Autodesk Inventor part; units mm, degrees
ref_plane "YZ Plane" through (0, 0, 0) normal (1, 0, 0) x (0, 1, 0)
ref_plane "XZ Plane" through (0, 0, 0) normal (0, 1, 0) x (-1, 0, 0)
ref_plane "XY Plane" through (0, 0, 0) normal (0, 0, 1) x (1, 0, 0)
sketch "Sketch1" plane through (0, 0, 0) normal (0, 0, 1) x (1, 0, 0)
  circle A0 centre (0, 0) radius 17.5
  line L0 (14.8492, -14.8492) -> (-14.8492, -14.8492) construction
  line L1 (-14.8492, -14.8492) -> (-14.8492, 14.8492) construction
  line L2 (-14.8492, 14.8492) -> (14.8492, 14.8492) construction
  line L3 (14.8492, 14.8492) -> (14.8492, -14.8492) construction
  line L4 (14.8492, -14.8492) -> (-14.8492, 14.8492) construction
  line L5 (-14.8492, -14.8492) -> (14.8492, 14.8492) construction
  circle A1 centre (0, 0) radius 21 construction
  line L6 (21, -21) -> (-21, -21) construction
  line L7 (-21, -21) -> (-21, 21) construction
  line L8 (-21, 21) -> (21, 21) construction
  line L9 (21, 21) -> (21, -21) construction
  line L10 (21, -21) -> (-21, 21) construction
  line L11 (-21, -21) -> (21, 21) construction
  line L12 (-31.85, -21.15) -> (-74.15, -21.15) construction
  line L13 (-74.15, -21.15) -> (-74.15, 21.15) construction
  line L14 (-74.15, 21.15) -> (-31.85, 21.15) construction
  line L15 (-31.85, 21.15) -> (-31.85, -21.15) construction
  line L16 (-31.85, -21.15) -> (-74.15, 21.15) construction
  line L17 (-74.15, -21.15) -> (-31.85, 21.15) construction
  line L18 (-37.5, -15.5) -> (-68.5, -15.5) construction
  line L19 (-68.5, -15.5) -> (-68.5, 15.5) construction
  line L20 (-68.5, 15.5) -> (-37.5, 15.5) construction
  line L21 (-37.5, 15.5) -> (-37.5, -15.5) construction
  line L22 (-37.5, -15.5) -> (-68.5, 15.5) construction
  line L23 (-68.5, -15.5) -> (-37.5, 15.5) construction
  line L24 (-70.5, 15.5) -> (-66.5, 15.5) construction
  line L25 (-70.5, 13.85) -> (-66.5, 13.85)
  line L26 (-66.5, 17.15) -> (-70.5, 17.15)
  arc A2 (-70.5, 17.15) -> (-70.5, 13.85) centre (-70.5, 15.5) ccw
  arc A3 (-66.5, 13.85) -> (-66.5, 17.15) centre (-66.5, 15.5) ccw
  line L27 (-35.5, 15.5) -> (-39.5, 15.5) construction
  line L28 (-35.5, 17.15) -> (-39.5, 17.15)
  line L29 (-39.5, 13.85) -> (-35.5, 13.85)
  arc A4 (-35.5, 13.85) -> (-35.5, 17.15) centre (-35.5, 15.5) ccw
  arc A5 (-39.5, 17.15) -> (-39.5, 13.85) centre (-39.5, 15.5) ccw
  line L30 (-35.5, -15.5) -> (-39.5, -15.5) construction
  line L31 (-35.5, -13.85) -> (-39.5, -13.85)
  line L32 (-39.5, -17.15) -> (-35.5, -17.15)
  arc A6 (-35.5, -17.15) -> (-35.5, -13.85) centre (-35.5, -15.5) ccw
  arc A7 (-39.5, -13.85) -> (-39.5, -17.15) centre (-39.5, -15.5) ccw
  line L33 (-70.5, -15.5) -> (-66.5, -15.5) construction
  line L34 (-70.5, -17.15) -> (-66.5, -17.15)
  line L35 (-66.5, -13.85) -> (-70.5, -13.85)
  arc A8 (-70.5, -13.85) -> (-70.5, -17.15) centre (-70.5, -15.5) ccw
  arc A9 (-66.5, -17.15) -> (-66.5, -13.85) centre (-66.5, -15.5) ccw
  line L36 (-55, 0) -> (-51, 0) construction
  line L37 (-55, -11.25) -> (-51, -11.25)
  line L38 (-51, 11.25) -> (-55, 11.25)
  arc A10 (-55, 11.25) -> (-55, -11.25) centre (-55, 0) ccw
  arc A11 (-51, -11.25) -> (-51, 11.25) centre (-51, 0) ccw
  line L39 (40, 54.25) -> (-40, 54.25) construction
  line L40 (-40, 54.25) -> (-40, 94.25) construction
  line L41 (-40, 94.25) -> (40, 94.25) construction
  line L42 (40, 94.25) -> (40, 54.25) construction
  line L43 (40, 54.25) -> (-40, 94.25) construction
  line L44 (-40, 54.25) -> (40, 94.25) construction
  line L45 (98.5, -30) -> (-98.5, -30)
  line L46 (-98.5, -30) -> (-98.5, 30)
  line L47 (-98.5, 30) -> (98.5, 30)
  line L48 (98.5, 30) -> (98.5, -30)
  line L49 (98.5, -30) -> (-98.5, 30) construction
  line L50 (-98.5, -30) -> (98.5, 30) construction
  line L51 (-77, 22) -> (-29, 22)
  line L52 (-29, 22) -> (-29, -22)
  line L53 (-29, -22) -> (-77, -22)
  line L54 (-77, -22) -> (-77, 22)
  line L55 (-77, 22) -> (-29, -22) construction
  line L56 (-29, 22) -> (-77, -22) construction
  line L57 (80, 30) -> (100, 30) construction
  line L58 (100, 30) -> (100, -30) construction
  line L59 (100, -30) -> (80, -30) construction
  line L60 (80, -30) -> (80, 30) construction
  line L61 (80, 30) -> (100, -30) construction
  line L62 (100, 30) -> (80, -30) construction
  line L63 (-80, 30) -> (-100, 30) construction
  line L64 (-100, 30) -> (-100, -30) construction
  line L65 (-100, -30) -> (-80, -30) construction
  line L66 (-80, -30) -> (-80, 30) construction
  line L67 (-80, 30) -> (-100, -30) construction
  line L68 (-100, 30) -> (-80, -30) construction
  line L69 (-83, -28) -> (-23, -28) construction
  line L70 (-23, -28) -> (-23, 28) construction
  line L71 (-23, 28) -> (-83, 28) construction
  line L72 (-83, 28) -> (-83, -28) construction
  circle A12 centre (0, 0) radius 34 construction
  line L73 (-28, -28) -> (28, -28) construction
  line L74 (28, -28) -> (28, 28) construction
  line L75 (28, 28) -> (-28, 28) construction
  line L76 (-28, 28) -> (-28, -28) construction
  line L77 (-28, -28) -> (28, 28) construction
  line L78 (28, -28) -> (-28, 28) construction
  circle A13 centre (0, 0) radius 25 construction
  line L79 (0, 0) -> (9.5671, 23.097) construction
  point P0 (-53, 0)
  point P1 (0, 74.25)
  point P2 (90, 0)
  point P3 (-90, 0)
  dimension "d1" = 42
  dimension "d44" = 50
  dimension "d0" = 35
  dimension "d2" = 42
  dimension "d3" = 42
  dimension "d4" = 42.3
  dimension "d5" = 42.3
  dimension "d6" = 53
  dimension "d7" = 31
  dimension "d8" = 31
  dimension "d9" = 1.65
  dimension "d10" = 4
  dimension "d11" = 11.25
  dimension "d12" = 80
  dimension "d13" = 40
  dimension "d14" = 54.25
  dimension "d15" = 197
  dimension "d16" = 60
  dimension "d35" = 48
  dimension "d36" = 44
  dimension "d37" = 20
  dimension "d38" = 90
  dimension "d39" = 90
  dimension "d40" = 6
  dimension "d41" = 68
  dimension "d42" = 56
  dimension "d43" = 56
  dimension "d45" = 22.5
extrude "Extrusion1" add sketch "Sketch1" along normal blind 6.35 contours L45 L46 L47 L48 | L51 L52 L53 L54
hole "Hole3" at (14.8492, 14.8492, 0) at (-14.8492, 14.8492, 0) at (14.8492, -14.8492, 0) at (-14.8492, -14.8492, 0) direction (0, 0, 1) diameter 3.242 end through all
sketch "Sketch2" plane through (0, 0, 6.35) normal (0, 0, 1) x (1, 0, 0)
  line L0 (90, -21.5) -> (-90, -21.5) construction
  line L1 (-90, -21.5) -> (-90, 21.5) construction
  line L2 (-90, 21.5) -> (90, 21.5) construction
  line L3 (90, 21.5) -> (90, -21.5) construction
  line L4 (90, -21.5) -> (-90, 21.5) construction
  line L5 (-90, -21.5) -> (90, 21.5) construction
  line L6 (98.5, 30) -> (-98.5, 30) construction
  line L7 (-98.5, 30) -> (-90, 30) construction
  line L8 (-90, 30) -> (-90, 21.5) construction
  line L9 (-90, 21.5) -> (-98.5, 21.5) construction
  line L10 (-98.5, 21.5) -> (-98.5, 30) construction
  point P0 (0, 0)
  point P1 (-90, 0)
  point P2 (90, 0)
  dimension "d26" = 180
hole "Hole2" at (-90, 0, 6.35) at (-90, 21.5, 6.35) at (-90, -21.5, 6.35) at (90, 21.5, 6.35) at (90, 0, 6.35) at (90, -21.5, 6.35) direction (0, 0, -1) diameter 5.3 end through all
fillet "Fillet1" radius 2 4 edges at (-98.5, -30, 3.175) (-98.5, 30, 3.175) (98.5, 30, 3.175) (98.5, -30, 3.175)
sketch "Sketch3" plane through (0, 0, 0) normal (0, 0, -1) x (-1, 0, 0)
  line L0 (53, 0) -> (-53, 0) construction
  line L1 (-43, -10) -> (-63, -10) construction
  line L2 (-63, -10) -> (-63, 10) construction
  line L3 (-63, 10) -> (-43, 10) construction
  line L4 (-43, 10) -> (-43, -10) construction
  line L5 (-43, -10) -> (-63, 10) construction
  line L6 (-63, -10) -> (-43, 10) construction
  circle A0 centre (-53, 0) radius 7.5
  point P0 (0, 0)
  point P1 (0, 0)
  dimension "d56" = 20
  dimension "d57" = 20
  dimension "d58" = 15
extrude "Extrusion2" cut sketch "Sketch3" against normal through all
hole "Hole4" at (-53, 0, 0) at (63, 10, 0) at (43, 10, 0) at (43, -10, 0) at (63, -10, 0) direction (0, 0, 1) diameter 3.3 end through all
equation "\"d35\" = d36 + d10"
properties part number "Z-Axis Drive Mount RevII" material "Aluminum 6061"
Work out the finished part from the listing and answer in its coordinate system (mm). A direction names the side the tool comes from. Round coordinates to 2 decimals unless told otherwise and drop trailing zeros. Order: outer loops, then holes, each group sorted by start corner. A loop starts at its lowest first (then second) coordinate and runs counter-clockwise, first axis right, second up. Notation, with made-up numbers: M 28.5,5 L 70.5,5 A6 cw 70.5,13 Z; hole C 19,8 d2. An arc over 180 degrees is marked long. Put each result on its own line as item: value. Start each with the question number.
Q1. Section A-A, the plane y = 0 is taken. Write down the section's boundary in (x, z), and give its area (3 significant figures).
Q2. A tool of negligible diameter and unlimited length cuts with its end or side. For faces 1 (the cylindrical face through (-64.85, 15.54, 3.13)), 2 (the flat face through (98.5, 0, 3)), from which of +Z, -Z, +X, -X, +Y, -Y can it reach the whole face along a straight path? Write none if from no direction.
Q3. Section D-D, the plane y = 21.5 is taken. Write down the section's boundary in (x, z).
Q4. Section B-B, the plane x = 90 is taken. Write down the section's boundary in (y, z).
Q5. For a pull along Y with two mould halves and no side action, classify faces 3 (the flat face through (-1, 30, 3)), 4 (the flat face through (1, -30, 3)), 5 (the cylindrical face through (-13.41, -14.1, 3.22)) as pulls with the +Y half, pulls with the -Y half, needs draft (parallel to the pull), parting line crosses it, or undercut.
Q6. Straight lines are drawn through the part: L1, parallel to Y at x = 63, z = 4.75; L2, parallel to X at y = 21.5, z = 3.5; L3, parallel to X at y = 5, z = 0.75. For each, find the intervals that lie inside material, in ascending order. Write a range as [from, to].
Q7. Section C-C, the plane x = 43 is taken. Write down the section's boundary in (y, z).
Findings below:
1. outline: M -98.5,0 L -92.65,0 L -92.65,6.35 L -98.5,6.35 Z; M -87.35,0 L -66.25,0 L -66.25,6.35 L -87.35,6.35 Z; M -39.75,0 L -17.5,0 L -17.5,6.35 L -39.75,6.35 Z; M 17.5,0 L 45.5,0 L 45.5,6.35 L 17.5,6.35 Z; M 60.5,0 L 87.35,0 L 87.35,6.35 L 60.5,6.35 Z; M 92.65,0 L 98.5,0 L 98.5,6.35 L 92.65,6.35 Z
1. area: 698 mm^2
2. face 1: +Z, -Z
2. face 2: +Z, -Z, +X, +Y, -Y
3. outline: M -98.5,0 L -92.65,0 L -92.65,6.35 L -98.5,6.35 Z; M -87.35,0 L 87.35,0 L 87.35,6.35 L -87.35,6.35 Z; M 92.65,0 L 98.5,0 L 98.5,6.35 L 92.65,6.35 Z
4. outline: M -30,0 L -24.15,0 L -24.15,6.35 L -30,6.35 Z; M -18.85,0 L -2.65,0 L -2.65,6.35 L -18.85,6.35 Z; M 2.65,0 L 18.85,0 L 18.85,6.35 L 2.65,6.35 Z; M 24.15,0 L 30,0 L 30,6.35 L 24.15,6.35 Z
5. face 3: pulls with the +Y half
5. face 4: pulls with the -Y half
5. face 5: undercut
6. L1: y = [-30, -11.65], [-8.35, 8.35], [11.65, 30]
6. L2: x = [-98.5, -92.65], [-87.35, 87.35], [92.65, 98.5]
6. L3: x = [-98.5, -65.08], [-40.92, -16.77], [16.77, 47.41], [58.59, 98.5]
7. outline: M -30,0 L -11.65,0 L -11.65,6.35 L -30,6.35 Z; M -8.35,0 L 8.35,0 L 8.35,6.35 L -8.35,6.35 Z; M 11.65,0 L 30,0 L 30,6.35 L 11.65,6.35 Z
